```python
from build123d import *

# Parameters (mm, degrees)
F0_W     = 72.842926
F0_H     = 53.87415
F1_DEPTH = 25.4
F2_R     = 12.415196
F3_DEPTH = 25.4
F5_DEPTH = 40.132


with BuildPart() as f1:
    # F0 (on Front) → F1 (new body)
    with BuildSketch(Plane.XZ):
        with Locations((36.421463, -26.937075)):
            Rectangle(F0_W, F0_H)
    extrude(amount=F1_DEPTH)

    # F2 (on face) → F3 (join)
    with BuildSketch(Plane(origin=(0, 0, 0), x_dir=(-1, 0, 0), z_dir=(0, 1, 0))):
        with Locations((-41.560825, -19.02597)):
            Circle(F2_R)
    extrude(amount=F3_DEPTH)

    # F4 (on Top) → F5 (cut)
    with BuildSketch(Plane.XY):
        Polygon((61.878242, 30.363508), (18.419566, 24.895199), (61.878242, 10.792716), align=None)
    extrude(amount=-F5_DEPTH, mode=Mode.SUBTRACT)


solid = f1.part
```
Work out the finished part from the listing and answer in its coordinate system (mm). A direction names the side the tool comes from. Give positions to 0.01 mm unless a question says otherwise; leave off trailing zeros. Order: outer loops, then holes, each group sorted by start corner. A loop starts at its lowest first (then second) coordinate and runs counter-clockwise, first axis right, second up.
1. Section A-A, the plane x = 66.5 is taken. Determine the outline of the cut face in (y, z).
Result sheet:
outline: (-25.4, -53.87) - (0, -53.87) - (0, 0) - (-25.4, 0) - close
2. Each of these flat-tipped pins is pushed along its axis until it touches: P1, Ø8, axis at x = 60.5, z = -43.5, coming from the +Y side; P2, Ø6, axis at y = 12, z = -20, coming from the -X side; P3, Ø12, axis at y = 11.5, z = -25.5, coming from the +X side. Where does it stop, or does it pass through?
Result sheet:
P1: stops at y = 0
P2: stops at x = 29.15
P3: stops at x = 53.97
3. Section B-B, the plane z = -8 is taken. Determine the outline of the cut face in (x, y), and give its area (3 significant figures).
Result sheet:
outline: (0, -25.4) - (72.84, -25.4) - (72.84, 0) - (47.27, 0) - (47.27, 15.53) - (35.85, 19.24) - (35.85, 0) - (0, 0) - close
area: 2,050 mm2
4. Section C-C, the plane y = 4.5 is taken. Determine the outline of the cut face in (x, z).
Result sheet:
outline: circle Ø24.83 at (41.56, -19.03)
5. For faces 1 (the flat face through (41.39, 17.44, -18.85)), 2 (the cylindrical face through (29.72, 8.18, -15.3)), determine the directions among +Z, -Z, +X, -X, +Y, -Y from which every point of the face is accessible in a straight line to the end or side of a thin tool.
Result sheet:
face 1: +Z, -Z, +X, +Y
face 2: +Y
6. Straight lines are drawn through the part: L1, parallel to Y at x = 65, z = -9; L2, parallel to Z at x = 45, y = 4; L3, parallel to X at y = 2, z = -29. For each, find the intervals that lie inside material, in ascending order.
Result sheet:
L1: y = -25.4 to 0
L2: z = -30.96 to -7.1
L3: x = 34.17 to 48.95
7. Section D-D, the plane x = 37.5 is taken. Determine the outline of the cut face in (y, z).
Result sheet:
outline: (-25.4, -53.87) - (0, -53.87) - (0, -30.76) - (18.7, -30.76) - (18.7, -7.29) - (0, -7.29) - (0, 0) - (-25.4, 0) - close
